Model file for the job. Use its own axes, mm. A direction names the side the tool comes from. Coordinates: 2 decimals unless noted, no trailing zeros. Write each loop counter-clockwise with the first axis right and the second up, starting at its lowest first coordinate (ties: lowest second). Pieces come first, ordered by that corner, then holes. Notation, with made-up numbers: (37.5, 13) - (87.5, 13) arc R19 cw to (87.5, 21) - close; hole circle Ø5 at (89.25, 68.5). An arc over 180 degrees is marked (long way). Put each result on its own line as item: value. Start each with the question number.
1. Drill centre lines: L1, parallel to Y at x = -5, z = -6; L2, parallel to X at y = 3, z = -23; L3, parallel to X at y = 2.75, z = -4. Where is each one in solid material? Low to high. Write a range as from..to.
2. Saw through at D-D, the plane x = -51. Write the cut outline in (y, z).
3. Saw through at A-A, the plane x = -5.08. Give the number of separate pieces and of enclosed holes in the cut face, plus the area to 3 significant figures.
4. Saw through at C-C, the plane z = -13. Write the cut outline in (x, y), plus the area to 3 significant figures.
5. Pull direction X, two halves, no side cores. Call faces 4 (the face through (-3.81, 3.23, -4.16)), 5 (the face through (-60.18, 3.22, -30.61)), 6 (the face through (-44, 6.35, -18)), 7 (the face through (-3.81, 3.23, -34.71)): released by +X, released by -X, zero draft, split by the parting line, or undercut.
6. Which spindle directions (+Z, -Z, +X, -X, +Y, -Y) get a long thin tool onto all of the face, cutting with end or side? Do faces 1 (the face through (-4, 2, -8.446)), 2 (the face through (-62.591, 3.219, 1.184)), 3 (the face through (-79, 3, -2.07)). Say none if no direction does.
7. Drop flat-ended pins along their axis: P1, Ø1.5, axis at x = -80.55, y = 3.18, coming from the +Z side; P2, Ø1, axis at y = 2, z = -12.5, coming from the +X side; P3, Ø1, axis at x = -54, y = 4.5, coming from the +Z side; P4, Ø3, axis at x = -80.55, y = 3.18, coming from the -Z side. Give the stop position or say it passes through.
```python
from build123d import *

# Parameters (mm, degrees)
BOSS_EXTRUDE1_DEPTH     = 6.35
CUT_EXTRUDE2_DEPTH      = 95.416035655
CUT_EXTRUDE2_DEPTH_BACK = 95.416035655
SKETCH2_R               = 1.27
CUT_EXTRUDE5_DEPTH      = 95.965858186
CUT_EXTRUDE7_DEPTH      = 25.4
SKETCH6_W               = 10.4785697
SKETCH6_H               = 6.35
SKETCH6_R               = 1.0795
BOSS_EXTRUDE2_DEPTH     = 12.7
FILLET5_R               = 12.7
FILLET6_R               = 5.08
BOSS_EXTRUDE3_DEPTH     = 6.35
SKETCH10_R              = 1.2065
CUT_EXTRUDE9_DEPTH      = 94.912222776
SKETCH12_W              = 15.691210344
SKETCH12_H              = 20.701
CUT_EXTRUDE10_DEPTH     = 95.965858193


with BuildPart() as part:
    # Sketch1 → Boss-Extrude1 (new body)
    with BuildSketch(Plane(origin=(0, 0, 0), x_dir=(1, 0, 0), z_dir=(0, 1, 0))):
        Polygon((0, 0), (0, 38.989), (-10.16, 38.989), (-71.628, 29.4386), (-86.36, 29.4386), (-86.36, -4.5974), (-76.2, -4.5974), (-10.16, 0), align=None)
    extrude(amount=BOSS_EXTRUDE1_DEPTH)

    # Sketch2 → Cut-Extrude2 (cut, two sides: drawn at the far end of the back side and taken through both)
    with BuildSketch(Plane(origin=(-0.604981675, 0, 0), x_dir=(-1, 0, 0), z_dir=(0, 0, -1)).offset(-CUT_EXTRUDE2_DEPTH_BACK)):
        with Locations((4.475018325, 3.175)):
            Circle(SKETCH2_R)
        with Locations(Location((79.949388362, 3.175, 0), (0, 0, 180))):
            Circle(SKETCH2_R)
    extrude(amount=CUT_EXTRUDE2_DEPTH + CUT_EXTRUDE2_DEPTH_BACK, mode=Mode.SUBTRACT)

    # Sketch3 → Cut-Extrude5 (cut, through all)
    with BuildSketch(Plane(origin=(0, 0, 0), x_dir=(1, 0, 0), z_dir=(0, 1, 0))):
        with BuildLine():
            Line((-81.915, 22.7711), (-71.755, 22.7711))
            Line((-71.755, 22.7711), (-58.487579402, 20.207642468))
            ThreePointArc((-58.487579402, 20.207642468), (-55.580114305, 14.192748547), (-57.777398298, 7.883687982))
            Line((-57.777398298, 7.883687982), (-71.755, 2.0701))
            Line((-71.755, 2.0701), (-81.915, 2.0701))
            Line((-81.915, 2.0701), (-81.915, 22.7711))
        make_face()
        with BuildLine():
            Line((0, 30.5435), (0, 8.4455))
            Line((0, 8.4455), (-7.9756, 8.4455))
            Line((-7.9756, 8.4455), (-17.739567161, 7.096263095))
            Line((-17.739567161, 7.096263095), (-24.764375431, 7.587485542))
            ThreePointArc((-24.764375431, 7.587485542), (-25.820245836, 7.814780317), (-26.769908004, 8.32923828))
            ThreePointArc((-26.769908004, 8.32923828), (-31.345543526, 16.545378703), (-28.210906636, 25.41191441))
            ThreePointArc((-28.210906636, 25.41191441), (-27.55579932, 25.957953915), (-26.795645997, 26.34459543))
            Line((-26.795645997, 26.34459543), (-15.585156538, 30.5435))
            Line((-15.585156538, 30.5435), (-7.9756, 30.5435))
            Line((-7.9756, 30.5435), (0, 30.5435))
        make_face()
    extrude(amount=CUT_EXTRUDE5_DEPTH, mode=Mode.SUBTRACT)

    # Sketch5 → Cut-Extrude7 (cut)
    with BuildSketch(Plane(origin=(0, 6.35, 0), x_dir=(1, 0, 0), z_dir=(0, 1, 0))):
        Polygon((-10.16, 38.989), (-53.78735915, 28.179846815), (-71.628, 29.4386), align=None)
        Polygon((-10.16, 0), (-47.394119509, 2.627067431), (-76.2, -4.5974), align=None)
    extrude(amount=-CUT_EXTRUDE7_DEPTH, mode=Mode.SUBTRACT)

    # Sketch6 → Boss-Extrude2 (add)
    with BuildSketch(Plane.XY.offset(-31.75)):
        with Locations((-43.810886798, 3.175)):
            Rectangle(SKETCH6_W, SKETCH6_H)
        with Locations((-45.72, 3.108706623)):
            Circle(SKETCH6_R, mode=Mode.SUBTRACT)
        with Locations((-42.164, 3.108706623)):
            Circle(SKETCH6_R, mode=Mode.SUBTRACT)
    extrude(amount=BOSS_EXTRUDE2_DEPTH)

    # Fillet5
    fillet5_edges = [part.edges().sort_by_distance(p)[0] for p in [
        (-47.394119509, 3.175, -2.627067431),
        (-53.78735915, 3.175, -28.179846815),
    ]]
    fillet(fillet5_edges, radius=FILLET5_R)

    # Fillet6
    fillet6_edges = [part.edges().sort_by_distance(p)[0] for p in [
        (-57.777398298, 3.175, -7.883687982),
        (-58.487579402, 3.175, -20.207642468),
    ]]
    fillet(fillet6_edges, radius=FILLET6_R)

    # Sketch9 → Boss-Extrude3 (add)
    with BuildSketch(Plane(origin=(0, 6.35, 0), x_dir=(1, 0, 0), z_dir=(0, 1, 0))):
        Polygon((-49.050171648, 31.75), (-71.628, 29.4386), (-71.628, 26.697361781), (-49.050171648, 26.697361781), align=None)
    extrude(amount=-BOSS_EXTRUDE3_DEPTH)

    # Sketch10 → Cut-Extrude9 (cut, through all)
    with BuildSketch(Plane(origin=(0, 0, -31.75), x_dir=(-1, 0, 0), z_dir=(0, 0, -1))):
        with Locations((42.164, 3.108706623)):
            Circle(SKETCH10_R)
        with Locations((45.72, 3.108706623)):
            Circle(SKETCH10_R)
    extrude(amount=-CUT_EXTRUDE9_DEPTH, mode=Mode.SUBTRACT)

    # Sketch12 → Cut-Extrude10 (cut, through all)
    with BuildSketch(Plane(origin=(0, 0, 0), x_dir=(1, 0, 0), z_dir=(0, 1, 0))):
        with Locations((-89.760605172, 12.4206)):
            Rectangle(SKETCH12_W, SKETCH12_H)
    extrude(amount=CUT_EXTRUDE10_DEPTH, mode=Mode.SUBTRACT)


solid = part.part
```
Final values:
1. L1: y = 0..1.91, 4.44..6.35
1. L2: x = -86.36..-81.81, -79.3..-46.92, -44.52..-43.37, -40.96..-29.98
1. L3: x = -67.11..-46.87, -44.57..-43.32, -41.01..-6.28, -3.88..0
2. outline: (0, -31.55) - (6.35, -31.55) - (6.35, -1.72) - (0, -1.72) - close
3. separate pieces: 4
3. enclosed holes: 0
3. area: 64.4 mm²
4. outline: (-55.59, 0) - (-30.46, 0) - (-30.46, 6.35) - (-55.59, 6.35) - close; hole circle Ø2.41 at (-45.72, 3.11); hole circle Ø2.41 at (-42.16, 3.11)
4. area: 150 mm²
5. face 4: undercut
5. face 5: released by -X
5. face 6: zero draft
5. face 7: undercut
6. face 1: +X, +Y, -Y
6. face 2: +Z, +Y, -Y
6. face 3: -X, +Y, -Y
7. P1: passes through
7. P2: stops at x = -29.97
7. P3: stops at z = -0.84
7. P4: stops at z = -29.44
